For this review, take the finished solid that the model builds, in its own axes (mm). Face numbers are marked on the shaded views. A direction names the side the tool comes from. Coordinates: 2 decimals unless noted, no trailing zeros. Write each loop counter-clockwise with the first axis right and the second up, starting at its lowest first coordinate (ties: lowest second). Pieces come first, ordered by that corner, then holes.
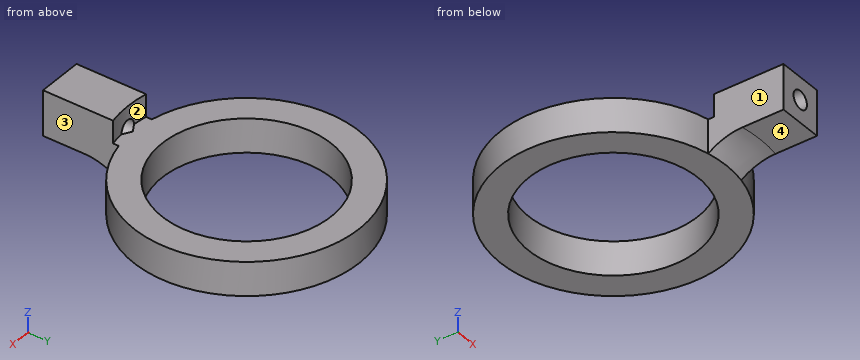
```python
from build123d import *

# Parameters (mm, degrees)
F0_R        = 10
F0_R_2      = 7.5
F1_DEPTH    = 3
F3_W        = 4
F3_H        = 7
F4_DEPTH    = 4
F5_R        = 10.5
F6_DEPTH    = 25
F7_T4_ANGLE = 109.021242163
F9_D        = 1.6
F9_DEPTH    = 6
F9_TIP      = 0.4806884952


# Not quite as in the source:
# - a fillet or chamfer that OpenCascade refuses, or shapes differently, is made with other operations: its cross-section is extruded or revolved along the edge and cut away or added


with BuildPart() as f1:
    # F0 (on Top) → F1 (new body)
    with BuildSketch(Plane.XY):
        Circle(F0_R)
        Circle(F0_R_2, mode=Mode.SUBTRACT)
    extrude(amount=F1_DEPTH)

    # F3 (on offset) → F4 (join)
    with BuildSketch(Plane.XY.offset(1)):
        with Locations((0.106652909, -13)):
            Rectangle(F3_W, F3_H)
    extrude(amount=F4_DEPTH)

    # F5 (on face) → F6 (cut)
    with BuildSketch(Plane.XY.offset(3)):
        Circle(F5_R)
    extrude(amount=F6_DEPTH, mode=Mode.SUBTRACT)

    # F7: fillet of radius 5 on 1 edges, made by hand


with BuildPart() as f7_tool2:
    # F7_s3 → F7_t4 (revolve)
    with BuildSketch(Plane(origin=(0, 0, 0), x_dir=(0, 0, 1), z_dir=(0.5716546179, 0.8204943618, 0))):
        with BuildLine():
            ThreePointArc((0, 10), (0.7434164903, 11.4188611699), (1, 13))
            Line((1, 13), (1, 10))
            Line((1, 10), (0, 10))
        make_face()
    revolve(axis=Axis((0, 0, 1), (0, 0, -1)), revolution_arc=F7_T4_ANGLE)

    split(bisect_by=Plane.YZ.offset(2.106652909), keep=Keep.BOTTOM)

    split(bisect_by=Plane.YZ.offset(-1.893347091), keep=Keep.TOP)


with BuildPart() as f1_1:
    add(f1.part)

    # F7_t1: union F7_tool2
    add(f7_tool2.part)

    # F9
    with Locations(Plane.XZ.offset(16.5)):
        with Locations((0.106652909, 3)):
            Hole(F9_D / 2, depth=F9_DEPTH)
            with Locations((0, 0, -(F9_DEPTH + F9_TIP / 2))):  # 118° drill point
                Cone(0, F9_D / 2, F9_TIP, mode=Mode.SUBTRACT)


solid = f1_1.part
```
Q1. Tool access review of the marked faces 1, 2, 3 and 4: name each direction out of +Z, -Z, +X, -X, +Y, -Y from which nothing blocks a thin tool from reaching the whole face with its end or side.
Ans:
face 1: +Z, -Z, -X, -Y
face 2: +Z, +Y
face 3: +Z, -Z, +X, -Y
face 4: -Z, +X, -X, -Y
Q2. Clearance check with flat-ended pins moving along their axes: pin 1 Ø1.5 at (y, z) = (-12, 2.5) entering from -X; pin 2 Ø10 at (x, y) = (4.5, 2.5) entering from +Z; pin 3 Ø1.8 at (x, y) = (0, -15) entering from -Z. State where each tip first meets the part, or that it passes through.
Ans:
pin 1: stops at x = -1.89
pin 2: stops at z = 3
pin 3: stops at z = 1
Q3. Add section B-B (x = -6). State the section outline as (y, z) points.
Ans:
outline: (-8, 0) - (-4.5, 0) - (-4.5, 3) - (-8, 3) - close; (4.5, 0) - (8, 0) - (8, 3) - (4.5, 3) - close
Q4. Add section A-A (y = 0). State the section outline as (x, z) points.
Ans:
outline: (-10, 0) - (-7.5, 0) - (-7.5, 3) - (-10, 3) - close; (7.5, 0) - (10, 0) - (10, 3) - (7.5, 3) - close
Q5. Add section C-C (x = 0.5). Give the number of separate pieces and of enclosed holes in the cut face, then the cut area to 3 significant figures.
Ans:
separate pieces: 3
enclosed holes: 0
area: 32.6 mm2
Q6. For probe 1 along X at (y, z) = (-13.35, 3); probe 2 along Y at (x, z) = (0, 1.1); probe 3 along Z at (x, y) = (7, -4.5), list the stretches that pass through material, from the lowest coordinate up.
Ans:
probe 1: x = -1.89 to -0.69, 0.91 to 2.11
probe 2: y = -16.5 to -7.5, 7.5 to 10
probe 3: z = 0 to 3
